Work out the finished part from the listing and answer in its coordinate system (mm). A direction names the side the tool comes from. Round coordinates to 2 decimals unless told otherwise and drop trailing zeros. Order: outer loops, then holes, each group sorted by start corner. A loop starts at its lowest first (then second) coordinate and runs counter-clockwise, first axis right, second up. Notation, with made-up numbers: (24, 15) - (38, 15) arc R32 cw to (38, 45) - close; hole circle Ø11 at (31, 62). An arc over 180 degrees is marked (long way). Answer in a Markdown table with one row per item.
from build123d import *

# Parameters (mm, degrees)
ESBO_O1_R                = 3
RESSALTO_EXTRUS_O1_DEPTH = 5


with BuildPart() as part:
    # Esboço1 → Ressalto-extrusão1 (new body)
    with BuildSketch(Plane.XY):
        Polygon((2.886751346, 5), (-2.886751346, 5), (-5.773502692, 0), (-2.886751346, -5), (2.886751346, -5), (5.773502692, 0), align=None)
        Circle(ESBO_O1_R, mode=Mode.SUBTRACT)
    extrude(amount=RESSALTO_EXTRUS_O1_DEPTH)

    # Esboço2 → Revolução1 (revolve)
    with BuildSketch(Plane(origin=(0, 0, 0), x_dir=(1, 0, 0), z_dir=(0, 1, 0))):
        with BuildLine():
            Line((0, 0), (5.273502692, 0))
            ThreePointArc((5.273502692, 0), (3.728929514, 3.728929514), (0, 5.273502692))
            Line((0, 5.273502692), (0, 0))
        make_face()
    revolve(axis=Axis((0, 0, -5.273502692), (0, 0, 1)))


solid = part.part
1) Which of the six approach directions +Z, -Z, +X, -X, +Y, -Y give full straight-line access (tool end or side, diameter ignored) to faces 1 (the face through (-4.35, -2.465, 2.465)), 2 (the face through (0, 0, 0)), 3 (the face through (-4.31, 2.535, 2.465)), 4 (the face through (-2.72, 4.71, 0))?
Filled in:
| item | result |
|---|---|
| face 1 | +Z, -X, -Y |
| face 2 | +Z |
| face 3 | +Z, -X, +Y |
| face 4 | -Z, -X, +Y |
2) The mould has two halves that part along X. Classify faces 5 (the face through (2.71, 4.71, 0)), 6 (the face through (-3, 0, 2)), 7 (the face through (4.35, 2.465, 2.465)): released by +X, released by -X, zero draft, split by the parting line, or undercut.
Filled in:
| item | result |
|---|---|
| face 5 | zero draft |
| face 6 | undercut |
| face 7 | released by +X |
3) Find section B-B, the plane x = 0. Give the vertices of the cut face in (y, z).
Filled in:
| item | result |
|---|---|
| outline | (-5.27, 0) arc R5.27 ccw to (5.27, 0) - (5, 0) - (5, 5) - (3, 5) - (3, 0) - (-3, 0) - (-3, 5) - (-5, 5) - (-5, 0) - close |
4) Find section D-D, the plane z = -4.5. Give the vertices of the cut face in (x, y).
Filled in:
| item | result |
|---|---|
| outline | circle Ø5.5 at (0, 0) |
5) Each of these flat-tipped pins is pushed along its axis until it touches: pin 1 (5.5 mm diameter, centred on x = -1, z = 3, fed in from -Y); pin 2 (0.8 mm diameter, centred on x = 2.5, y = -4.5, fed in from -Z); pin 3 (3 mm diameter, centred on y = -3.5, z = 0, fed in from -X). Where does it stop, or does it pass through?
Filled in:
| item | result |
|---|---|
| pin 1 | stops at y = -5 |
| pin 2 | stops at z = -2.3 |
| pin 3 | stops at x = -4.88 |
6) Find section C-C, the plane y = -2.75. Give the vertices of the cut face in (x, z), then the cut area to 3 significant figures.
Filled in:
| item | result |
|---|---|
| outline | (-4.5, 0) arc R4.5 ccw to (4.5, 0) - (4.19, 0) - (4.19, 5) - (1.2, 5) - (1.2, 0) - (-1.2, 0) - (-1.2, 5) - (-4.19, 5) - (-4.19, 0) - close |
| area | 61.7 mm^2 |
7) Find section A-A, the plane z = 3.75. Give the vertices of the cut face in (x, y).
Filled in:
| item | result |
|---|---|
| outline | (-5.77, 0) - (-2.89, -5) - (2.89, -5) - (5.77, 0) - (2.89, 5) - (-2.89, 5) - close; hole circle Ø6 at (0, 0) |
8) Find the intervals of material crossed by probe 1 along Y at (x, z) = (0, 1.65); probe 2 along X at (y, z) = (0.5, 4.5); probe 3 along X at (y, z) = (1, 2.25), in increasing order. Write a range as from..to.
Filled in:
| item | result |
|---|---|
| probe 1 | y = -5..-3, 3..5 |
| probe 2 | x = -5.48..-2.96, 2.96..5.48 |
| probe 3 | x = -5.2..-2.83, 2.83..5.2 |
